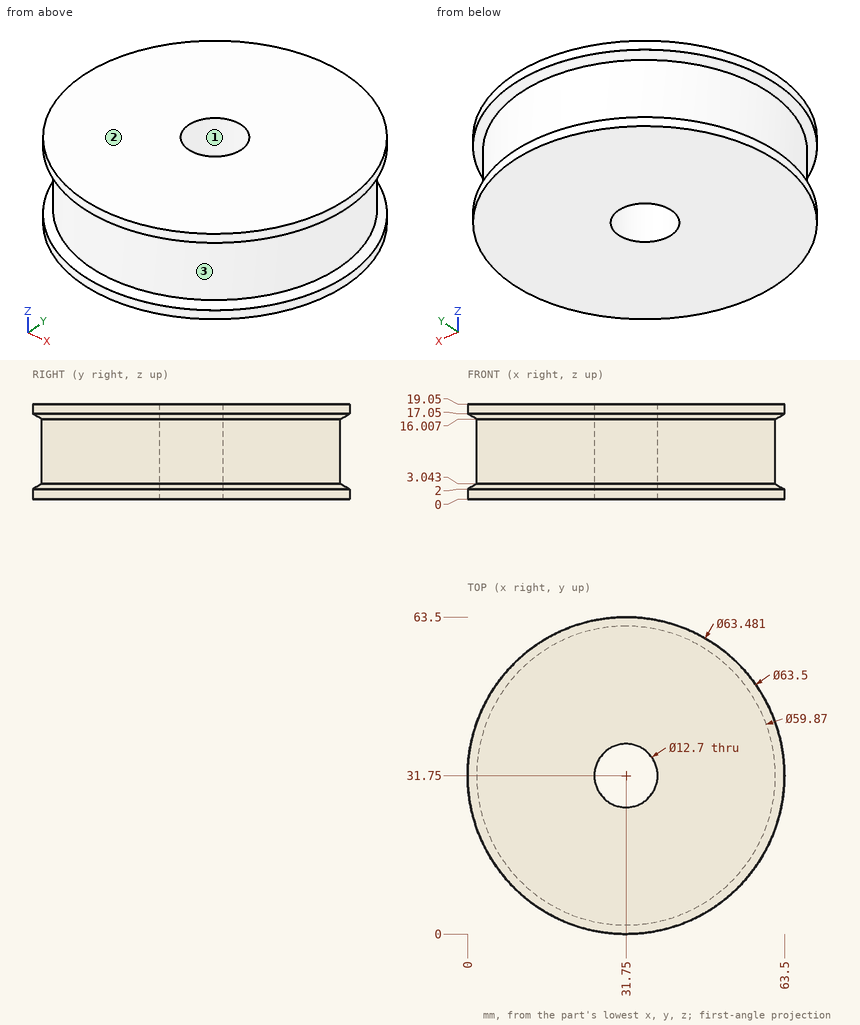
The figure shows three views and two pictorial views of one solid part (mm, origin at its lowest corner). Answer the questions. Round coordinates to 2 decimals unless told otherwise and drop trailing zeros. One line per question, with ' | ' between items. Start each with the question number.
Q1. Find the intervals of material crossed by L1, parallel to Y at x = 31.75, z = 8.25 (1 decimal); L2, parallel to X at y = 31.5, z = 16.75 (1 decimal); L3, parallel to Y at x = 36.5, z = 17.5 (1 decimal), in increasing order.
Q2. Flat-ended cylindrical pins translate along their axes: pin 1 (8 mm diameter, centred on x = 44, z = 11.5, fed in from +Y) (1 decimal); pin 2 (10 mm diameter, centred on x = 29.5, z = 6, fed in from -Y); pin 3 (6 mm diameter, centred on y = 14, z = 15.5, fed in from +X) (1 decimal). Find the tip coordinate at first contact, or state that the pin passes through.
Q3. For a pull along Y with two mould halves and no side action, classify the marked faces 1, 2 and 3 as +Y half, -Y half, draft (parallel to the pull), parting line (faces both ways), or undercut.
Established:
1) L1: 1.8 to 25.4, 38.1 to 61.7 | L2: 0.5 to 25.4, 38.1 to 63 | L3: 0.4 to 27.5, 36 to 63.1
2) pin 1: y = 60.5 | pin 2: y = 0 | pin 3: x = 59.6
3) face 1: undercut | face 2: draft | face 3: parting line
